Geometry check sheet. Reference: the model listing, model coordinates, mm. Give positions to 0.01 mm unless a question says otherwise; leave off trailing zeros. Loops run counter-clockwise (first coordinate to the right, second up) from the corner with the lowest first, then second, coordinate; pieces in that order, holes last. Notation, with made-up numbers: (-10.75, 16.5) -> (-2.75, 16.5) arc R18 ccw to (-2.75, 45.5) -> close; hole circle Ø5 at (31.5, 76.5). An arc over 180 degrees is marked (long way). Write item = value, one per line. Start each with the question number.
```python
from build123d import *

# Parameters (mm, degrees)
REDONDEO1_R = 1


with BuildPart() as part:
    # Croquis1 → Revolución1 (revolve)
    with BuildSketch(Plane.XY, mode=Mode.PRIVATE) as revoluci_n1_sk:
        Polygon((29.505177058, 0), (42.658761964, 129.1), (44, 129.1), (44, 132.5), (42, 132.5), (29.264150943, 7.5), (0, 7.5), (0, 6.5), (29.162264151, 6.5), (28.5, 0), align=None)
    revolve(revoluci_n1_sk.sketch.rotate(Axis((0, 0, 0), (0, 1, 0)), 90), axis=Axis((0, 0, 0), (0, 1, 0)))

    # Redondeo1
    redondeo1_edges = [part.edges().sort_by_distance(p)[0] for p in [
        (0, 132.5, 44),
        (0, 129.1, 44),
    ]]
    fillet(redondeo1_edges, radius=REDONDEO1_R)


solid = part.part
```
1) Section check C-C (y = 63). Enter the section's corners in (x, z), plus the area to 3 significant figures.
2) Draft check along Y on faces 1 (the flat face through (0, 7.5, 0)), 2 (the conical face through (25.31, 0.32, -13.17)), 3 (the conical face through (-10.87, 65.45, -34.5)), 4 (the cylindrical face through (42.954, 130.81, 9.538)). Enter one of: released by +Y, released by -Y, zero draft, split by the parting line, or undercut.
3) Section check D-D (y = 41.5). Enter the section's corners in (x, z).
4) Depth check by flat-ended pin: pin 1 Ø1 at (x, z) = (17, 21.5) entering from -Y; pin 2 Ø3 at (x, y) = (11, 14) entering from -Z; pin 3 Ø4 at (x, y) = (-2, 82.5) entering from +Z; pin 4 Ø2 at (x, z) = (32, 33) entering from -Y. Enter the tip coordinate at first touch or a pass-through.
5) Thickness scan on line 1 (X direction, y = 56, z = 30); line 2 (X direction, y = 97.5, z = -4.5); line 3 (Z direction, x = 28.5, y = 52). Record the ranges inside material, lowest first.
6) Section check A-A (z = 0). Enter the section's corners in (x, y).
7) Section check B-B (x = 0). Enter the section's corners in (y, z).
Check result:
q1.outline = circle Ø71.85 at (0, 0); hole circle Ø69.84 at (0, 0)
q1.area = 224 mm2
q2.face_1 = released by +Y
q2.face_2 = undercut
q2.face_3 = released by -Y
q2.face_4 = zero draft
q3.outline = circle Ø67.47 at (0, 0); hole circle Ø65.46 at (0, 0)
q4.pin_1 = 6.5
q4.pin_2 = -29.46
q4.pin_3 = 38.08
q4.pin_4 = through
q5.line_1 = -18.43 to -16.43, 16.43 to 18.43
q5.line_2 = -39.18 to -38.17, 38.17 to 39.18
q5.line_3 = -19.98 to -18.17, 18.17 to 19.98
q6.outline = (-44, 130.1) arc R1 ccw to (-43, 129.1) -> (-42.66, 129.1) -> (-29.51, 0) -> (-28.5, 0) -> (-29.16, 6.5) -> (29.16, 6.5) -> (28.5, 0) -> (29.51, 0) -> (42.66, 129.1) -> (43, 129.1) arc R1 ccw to (44, 130.1) -> (44, 131.5) arc R1 ccw to (43, 132.5) -> (42, 132.5) -> (29.26, 7.5) -> (-29.26, 7.5) -> (-42, 132.5) -> (-43, 132.5) arc R1 ccw to (-44, 131.5) -> close
q7.outline = (0, -29.51) -> (129.1, -42.66) -> (129.1, -43) arc R1 ccw to (130.1, -44) -> (131.5, -44) arc R1 ccw to (132.5, -43) -> (132.5, -42) -> (7.5, -29.26) -> (7.5, 29.26) -> (132.5, 42) -> (132.5, 43) arc R1 ccw to (131.5, 44) -> (130.1, 44) arc R1 ccw to (129.1, 43) -> (129.1, 42.66) -> (0, 29.51) -> (0, 28.5) -> (6.5, 29.16) -> (6.5, -29.16) -> (0, -28.5) -> close
